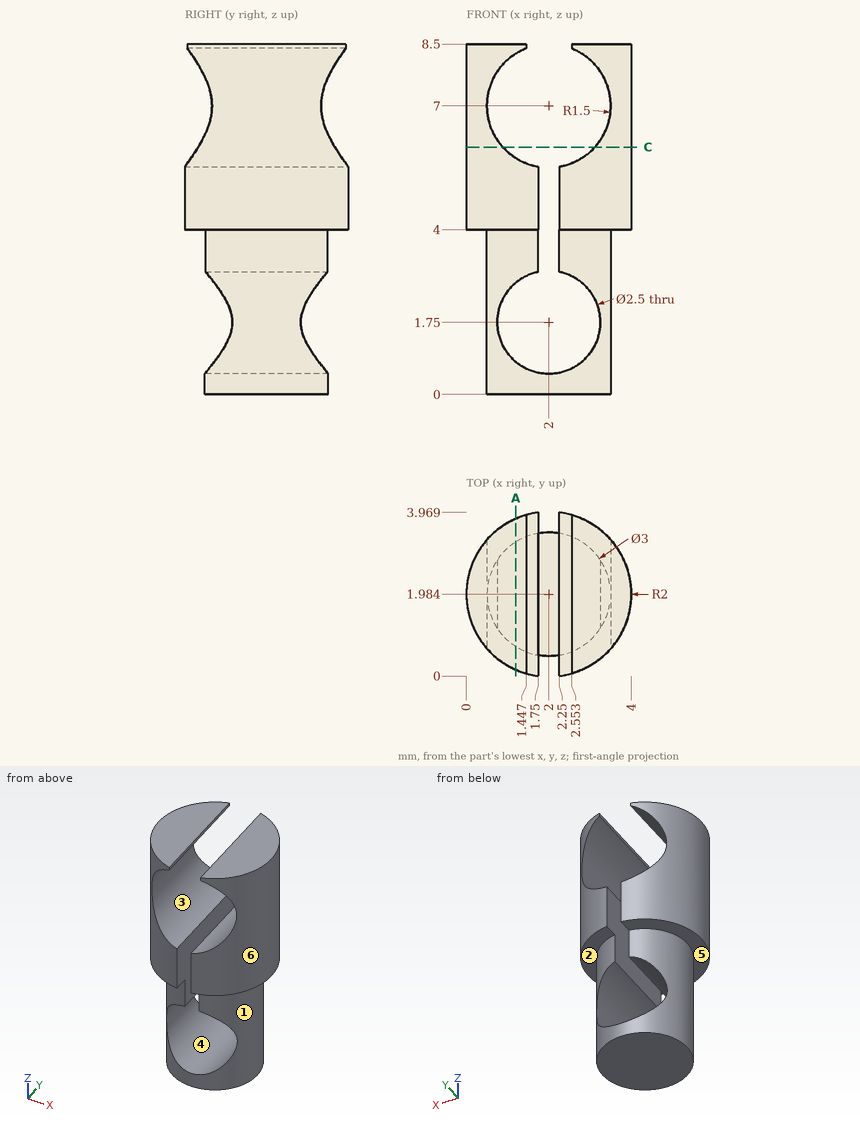
Answer from the drawing. Dimensions are ordinates in mm from the lowest x, y and z of the part. A direction names the side the tool comes from. Round coordinates to 2 decimals unless told otherwise and drop trailing zeros. Loops run counter-clockwise (first coordinate to the right, second up) from the corner with the lowest first, then second, coordinate; pieces in that order, holes last. Notation, with made-up numbers: (-17, -10) - (29, -10) arc R8 ccw to (29, -1) - close; hole circle Ø2 at (89.5, -25). An arc over 180 degrees is marked (long way). Return JSON: item names as keys, results as strings. Group by question number.
1. The part is cut by section A-A on x = 1.2. State how many separate pieces and enclosed holes the cut face has.
2. The part is cut by section C-C on z = 6. Determine the outline of the cut face in (x, y) (1 decimal).
3. This flat-tipped pin is pushed along its axis until it touches: P1, Ø2, axis at x = 2, z = 1.75, coming from the -Y side. Where does it stop, or does it pass through?
4. Which of the six approach directions +Z, -Z, +X, -X, +Y, -Y give full straight-line access (tool end or side, diameter ignored) to the marked faces 1, 2 and 3?
5. The mould has two halves that part along X. Classify the marked faces 4, 5 and 6: pulls with the +X half, pulls with the -X half, needs draft (parallel to the pull), parting line crosses it, or undercut.
6. Consider probe 1 along Z at (x, y) = (2, 2.4); probe 2 along Z at (x, y) = (3.1, 3.3); probe 3 along Z at (x, y) = (1.05, 2.1). Determine where each line is inside the solid, lowest interval first.
Resolved:
{
 "1": {"separate pieces": "3", "enclosed holes": "0"},
 "2": {"outline": "(0.9, 0.3) - (0.9, 3.6) arc R2 ccw to start; (3.1, 0.3) arc R2 ccw to (3.1, 3.6) - close"},
 "3": {"P1": "passes through"},
 "4": {"face 1": "-Z", "face 2": "-Z, +X", "face 3": "+Y, -Y"},
 "5": {"face 4": "undercut", "face 5": "needs draft", "face 6": "pulls with the +X half"},
 "6": {"probe 1": "z = 0 to 0.5", "probe 2": "z = 4 to 5.98, 8.02 to 8.5", "probe 3": "z = 0 to 0.94, 2.56 to 5.84, 8.16 to 8.5"}
}
